The drawing under review shows one solid part. Ordinate dimensions are in mm from its lowest x, y, z. A direction names the side the tool comes from. Coordinates: 2 decimals unless noted, no trailing zeros. Order: outer loops, then holes, each group sorted by start corner. A loop starts at its lowest first (then second) coordinate and runs counter-clockwise, first axis right, second up. Notation, with made-up numbers: M 5.25,-20 L 17.25,-20 A24 cw 17.25,11 Z; hole C 24.25,77 d9. An arc over 180 degrees is marked long. Answer as a JSON object with one key per item and string values.
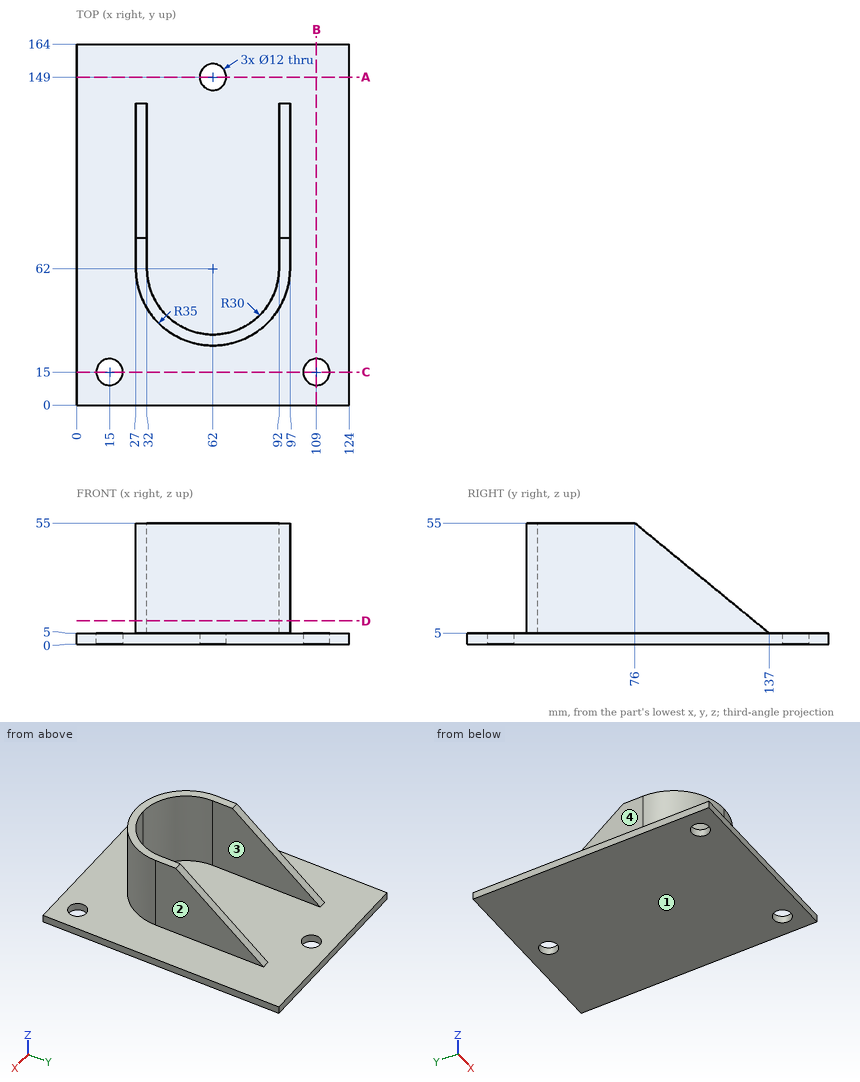
1) Add section B-B (x = 109). State the section outline as (y, z) points, and give its area (3 significant figures).
Taken from the geometry:
{"outline": "M 0,0 L 9,0 L 9,5 L 0,5 Z; M 21,0 L 164,0 L 164,5 L 21,5 Z", "area": "760 mm2"}
2) Tool access review of the marked faces 1, 2, 3 and 4: name each direction out of +Z, -Z, +X, -X, +Y, -Y from which nothing blocks a thin tool from reaching the whole face with its end or side.
Taken from the geometry:
{"face 1": "-Z, +X, -X, +Y, -Y", "face 2": "+Z, +X, +Y, -Y", "face 3": "+Z, +Y", "face 4": "+Z, -X, +Y, -Y"}
3) Add section D-D (z = 10.5). State the section outline as (x, y) points.
Taken from the geometry:
{"outline": "M 27,62 A35 ccw 97,62 L 97,130.29 L 92,130.29 L 92,62 A30 cw 32,62 L 32,130.29 L 27,130.29 Z"}
4) To check wall thickness, follow L1, parallel to X at y = 81, z = 21; L2, parallel to Y at x = 15, z = 1; L3, parallel to Y at x = 62, z = 1.5. State the ranges of each line that lie inside material, in increasing order.
Taken from the geometry:
{"L1": "x = 27 to 32, 92 to 97", "L2": "y = 0 to 9, 21 to 164", "L3": "y = 0 to 143, 155 to 164"}
5) Add section C-C (y = 15). State the section outline as (x, z) points, and give its area (3 significant figures).
Taken from the geometry:
{"outline": "M 0,0 L 9,0 L 9,5 L 0,5 Z; M 21,0 L 103,0 L 103,5 L 21,5 Z; M 115,0 L 124,0 L 124,5 L 115,5 Z", "area": "500 mm2"}
6) Add section A-A (y = 149). State the section outline as (x, z) points, and give its area (3 significant figures).
Taken from the geometry:
{"outline": "M 0,0 L 56,0 L 56,5 L 0,5 Z; M 68,0 L 124,0 L 124,5 L 68,5 Z", "area": "560 mm2"}
7) Insertion check: pin 1 Ø10 at (x, z) = (41, 23.5) entering from +Y; pin 2 Ø3 at (x, y) = (93.5, 109.5) entering from +Z; pin 3 Ø1.5 at (y, z) = (37.5, 12.5) entering from +X. Each pin has a flat end and moves straight along its axis. Give the tip position at first contact, or say it passes through.
Taken from the geometry:
{"pin 1": "stops at y = 47.03", "pin 2": "stops at z = 28.77", "pin 3": "stops at x = 87.71"}
